Input: dimensioned drawing with shaded views. Units: mm. Origin: part minimum x, y, z. A direction names the side the tool comes from. Coordinates: 2 decimals unless noted, no trailing zeros. Order: outer loops, then holes, each group sorted by start corner. A loop starts at its lowest first (then second) coordinate and runs counter-clockwise, first axis right, second up. Notation, with made-up numbers: M 12.25,44 L 25.25,44 A16 cw 25.25,52 Z; hole C 30.25,45 d1. An arc over 180 degrees is marked long. Use CSV: the item, a comma, the result in double quotes. Start each with the question number.
1. Section query B-B on z = 17.5. Return the cut outline in (x, y), and give its area (3 significant figures).
2. Pull-direction query (Z, two-part tool) for the marked faces 1, 2 and 3; classes: pulls with the +Z half, pulls with the -Z half, needs draft (parallel to the pull), parting line crosses it, or undercut.
3. Section query D-D on y = 3.25. Return the cut outline in (x, z), and give its area (3 significant figures).
4. Section query C-C on x = 45.5. Return the cut outline in (y, z), and give its area (3 significant figures).
5. Material intervals for line 1 (Z direction, x = 31, y = 10); line 2 (X direction, y = 10.5, z = 56); line 3 (Z direction, x = 38, y = 1.5), sorted ascending.
6. First-contact query: P1, Ø12, axis at x = 52.5, y = 11, coming from the +Z side; P2, Ø5, axis at x = 9.5, y = 6, coming from the -Z side; P3, Ø6, axis at y = 5, z = 110, coming from the +X side; P4, Ø1.5, axis at y = 5, z = 63.5, coming from the -X side. Flat tips, straight axial feed; report the tip coordinate or a pass-through.
7. Section query A-A on y = 10. Return the cut outline in (x, z), and give its area (3 significant figures).
8. Set-up query: the marked faces 4, 5, 6, 7 and 8. Return all of +Z, -Z, +X, -X, +Y, -Y with unobstructed straight access to the full face (end or side cutting, diameter ignored); none if empty.
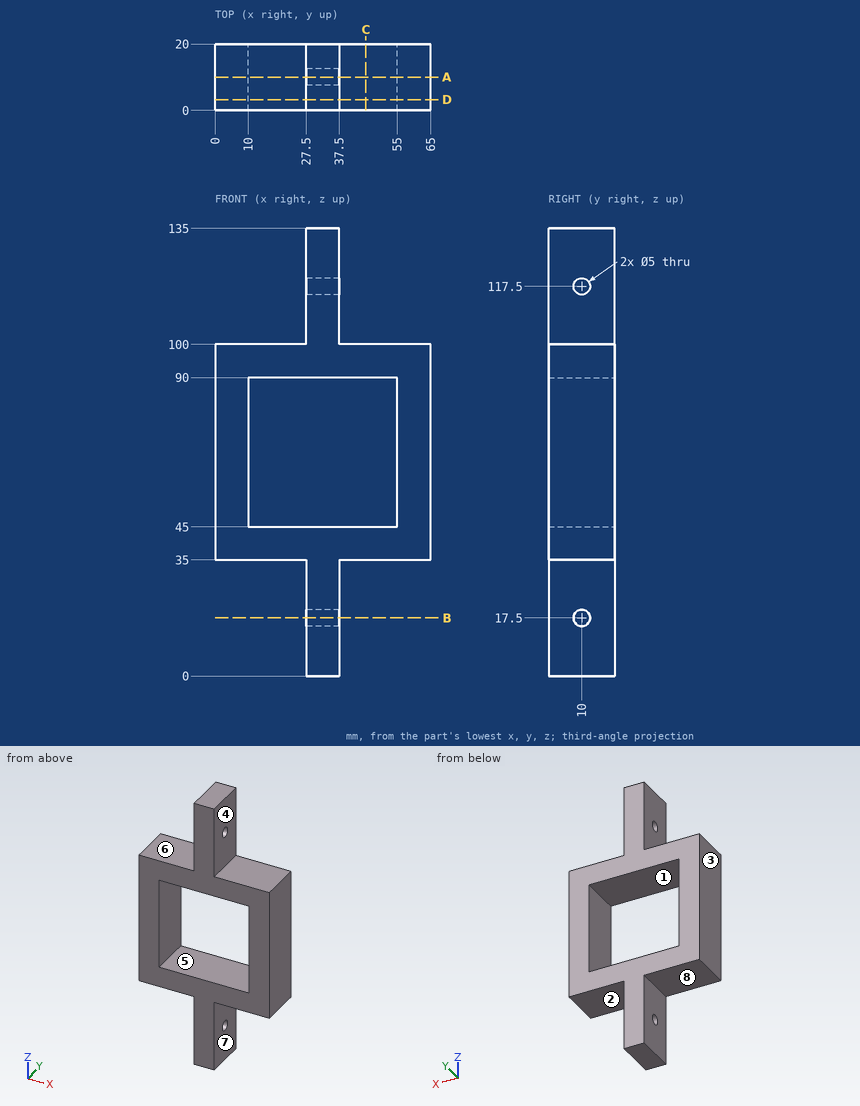
Results list:
1,outline,"M 27.5,0 L 37.5,0 L 37.5,7.5 L 27.5,7.5 Z; M 27.5,12.5 L 37.5,12.5 L 37.5,20 L 27.5,20 Z"
1,area,"150 mm²"
2,face 1,"undercut"
2,face 2,"pulls with the -Z half"
2,face 3,"needs draft"
3,outline,"M 0,35 L 27.5,35 L 27.5,0 L 37.5,0 L 37.5,35 L 65,35 L 65,100 L 37.5,100 L 37.5,135 L 27.5,135 L 27.5,100 L 0,100 Z; hole M 10,45 L 55,45 L 55,90 L 10,90 Z"
3,area,"2,900 mm²"
4,outline,"M 0,35 L 20,35 L 20,45 L 0,45 Z; M 0,90 L 20,90 L 20,100 L 0,100 Z"
4,area,"400 mm²"
5,line 1,"z = 0 to 15, 20 to 45, 90 to 115, 120 to 135"
5,line 2,"x = 0 to 10, 55 to 65"
5,line 3,"z = 35 to 45, 90 to 100"
6,P1,"stops at z = 100"
6,P2,"stops at z = 35"
6,P3,"stops at x = 37.5"
6,P4,"stops at x = 0"
7,outline,"M 0,35 L 27.5,35 L 27.5,20 L 37.5,20 L 37.5,35 L 65,35 L 65,100 L 37.5,100 L 37.5,115 L 27.5,115 L 27.5,100 L 0,100 Z; M 27.5,0 L 37.5,0 L 37.5,15 L 27.5,15 Z; M 27.5,120 L 37.5,120 L 37.5,135 L 27.5,135 Z; hole M 10,45 L 55,45 L 55,90 L 10,90 Z"
7,area,"2,800 mm²"
8,face 4,"+Z, +X, +Y, -Y"
8,face 5,"+Y, -Y"
8,face 6,"+Z, -X, +Y, -Y"
8,face 7,"-Z, +X, +Y, -Y"
8,face 8,"-Z, -X, +Y, -Y"
